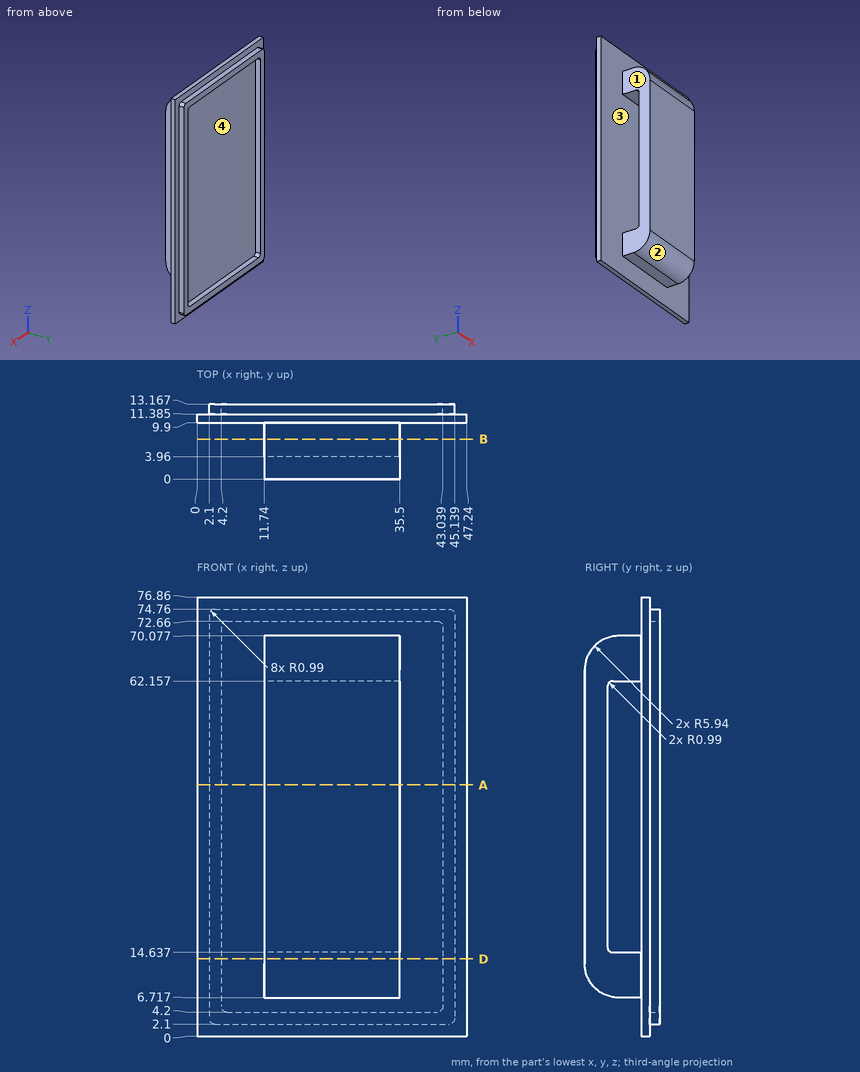
Drawing for the job (mm, zero at the part's lowest x, y, z). Round coordinates to 2 decimals unless told otherwise and drop trailing zeros. Order: outer loops, then holes, each group sorted by start corner. A loop starts at its lowest first (then second) coordinate and runs counter-clockwise, first axis right, second up.
Item 1: Mould opens along Y. For the marked faces 1, 2, 3 and 4 say: pulls with the +Y half, pulls with the -Y half, needs draft (parallel to the pull), parting line crosses it, or undercut.
Item 2: Probe line 1 along Y through (x, z) = (29, 16.5) (1 decimal); line 2 along Z through (x, y) = (38.5, 12.5); line 3 along Z through (x, y) = (22, 9.75). List the from-to ranges inside material, lowest first.
Item 3: Saw through at D-D on z = 13.5. Write the cut outline in (x, y) (1 decimal).
Item 4: Pin check, flat tips, straight feed: pin 1 (2 mm diameter, centred on x = 20, y = 7.5, fed in from +Z); pin 2 (2 mm diameter, centred on x = 14.5, y = 12, fed in from +Z); pin 3 (2 mm diameter, centred on y = 2.5, z = 25.5, fed in from -X); pin 4 (6 mm diameter, centred on x = 7.5, y = 6.5, fed in from -Z). Stop position of each tip, or through.
Item 5: Saw through at A-A on z = 44. Write the cut outline in (x, y) (1 decimal), then the cut area to 3 significant figures.
Item 6: Saw through at B-B on y = 7. Write the cut outline in (x, z).
Reported:
1. face 1: needs draft
1. face 2: pulls with the -Y half
1. face 3: undercut
1. face 4: pulls with the +Y half
2. line 1: y = 0 to 4, 9.9 to 11.4
2. line 2: z = 2.1 to 4.2, 72.66 to 74.76
2. line 3: z = 6.72 to 14.64, 62.16 to 70.08
3. outline: (0, 9.9) - (11.7, 9.9) - (11.7, 0) - (35.5, 0) - (35.5, 9.9) - (47.2, 9.9) - (47.2, 11.4) - (45.1, 11.4) - (45.1, 13.2) - (43, 13.2) - (43, 11.4) - (4.2, 11.4) - (4.2, 13.2) - (2.1, 13.2) - (2.1, 11.4) - (0, 11.4) - close
4. pin 1: stops at z = 70.08
4. pin 2: stops at z = 76.86
4. pin 3: stops at x = 11.74
4. pin 4: passes through
5. outline: (0, 9.9) - (47.2, 9.9) - (47.2, 11.4) - (45.1, 11.4) - (45.1, 13.2) - (43, 13.2) - (43, 11.4) - (4.2, 11.4) - (4.2, 13.2) - (2.1, 13.2) - (2.1, 11.4) - (0, 11.4) - close; (11.7, 0) - (35.5, 0) - (35.5, 4) - (11.7, 4) - close
5. area: 172 mm2
6. outline: (11.74, 6.72) - (35.5, 6.72) - (35.5, 14.64) - (11.74, 14.64) - close; (11.74, 62.16) - (35.5, 62.16) - (35.5, 70.08) - (11.74, 70.08) - close
